Autodesk Fusion 360 part; units mm, degrees
sketch "Sketch1" plane through (0, 0, 0) normal (0, 0, 1) x (1, 0, 0) in component "Some Fidget Keyboard"
  line L0 (0, 0) -> (42.54, 0)
  line L1 (42.54, 0) -> (42.54, 62.204)
  line L2 (42.54, 62.204) -> (0, 62.204)
  line L3 (0, 62.204) -> (0, 0)
  line L4 (-9.5, 72.704) -> (53.04, 72.704)
  line L5 (53.04, 72.704) -> (53.04, -9.5)
  line L6 (53.04, -9.5) -> (-9.5, -9.5)
  line L7 (-9.5, -9.5) -> (-9.5, 72.704)
  circle A0 centre (-4.5, 67.704) radius 1.7
  circle A1 centre (48.04, 67.704) radius 1.7
  circle A2 centre (48.04, -4.5) radius 1.7
  circle A3 centre (-4.5, -4.5) radius 1.7
  circle A4 centre (-4.5, 67.704) radius 3
  circle A5 centre (48.04, 67.704) radius 3
  circle A6 centre (48.04, -4.5) radius 3
  circle A7 centre (-4.5, -4.5) radius 3
  dimension "d4" = 42.54
  dimension "d5" = 62.204
  dimension "d6" = 62.54
  dimension "d7" = 82.204
  dimension "d8" = 9.5
  dimension "d9" = 9.5
  dimension "d10" = 3.4
  dimension "d11" = 3.4
  dimension "d12" = 3.4
  dimension "d13" = 3.4
  dimension "d14" = 5
  dimension "d15" = 5
  dimension "d16" = 5
  dimension "d17" = 5
  dimension "d18" = 5
  dimension "d20" = 5
  dimension "d21" = 5
  dimension "d22" = 5
  dimension "d23" = 6
  dimension "d24" = 6
  dimension "d25" = 6
  dimension "d26" = 6
extrude "Extrude1" add sketch "Sketch1" along normal blind 9.9 from surface at 3.1 contours A4 | A5 | A6 | A7 makes body 1 at (45.4801, 66.1397, 9.7) makes body 2 at (-7.0599, 66.1397, 9.7) makes body 3 at (51.0363, -4.6495, 9.7) makes body 4 at (-1.5037, -4.6495, 9.7) in component "Some Fidget Keyboard"
extrude "Extrude2" add sketch "Sketch1" along normal blind 13 contours L4 L5 L6 L7 bodies 1 2 3 4 in component "Some Fidget Keyboard"
extrude "Extrude3" add sketch "Sketch1" along normal blind 3 contours L0 L1 L2 L3 bodies 1 in component "Some Fidget Keyboard"
sketch "Sketch2" plane through (0, 0, 0) normal (0, 0, 1) x (1, 0, 0) in component "Some Fidget Keyboard"
sketch "Sketch3" plane through (0, 0, 13) normal (0, 0, 1) x (-1, 0, 0) in component "Some Fidget Keyboard"
  circle A0 centre (-48.04, -67.704) radius 1.7
  circle A1 centre (4.5, 4.5) radius 1.7
  line L0 (0, 0) -> (0, -62.204)
  line L1 (0, -62.204) -> (-42.54, -62.204)
  line L2 (-42.54, -62.204) -> (-42.54, 0)
  line L3 (-42.54, 0) -> (0, 0)
  line L4 (9.5, 9.5) -> (-53.04, 9.5)
  line L5 (-53.04, 9.5) -> (-53.04, -72.704)
  line L6 (-53.04, -72.704) -> (9.5, -72.704)
  line L7 (9.5, -72.704) -> (9.5, 9.5)
  circle A2 centre (4.5, -67.704) radius 1.7
  circle A3 centre (-48.04, 4.5) radius 1.7
  line L8 (-30.93, 9.5) -> (-12.43, 9.5)
  line L9 (-12.43, 9.5) -> (-12.43, 0)
  line L10 (-12.43, 0) -> (-30.93, 0)
  line L11 (-30.93, 0) -> (-30.93, 9.5)
  line L12 (-53.04, -72.704) -> (-53.04, 9.5)
  dimension "d36" = 18.5
  dimension "d37" = 22.11
extrude "Extrude4" cut sketch "Sketch3" against normal blind 7.5 contours L3 L4 L8 L9 L10 L11 bodies 1 in component "Some Fidget Keyboard"
fillet "Fillet1" radius 5 1 edges at (-9.5, -9.5, 6.5) on bodies 1 in component "Some Fidget Keyboard"
fillet "Fillet2" radius 5 1 edges at (-9.5, 72.704, 6.5) on bodies 1 in component "Some Fidget Keyboard"
fillet "Fillet3" radius 5 2 edges at (53.04, 72.704, 6.5) (53.04, -9.5, 6.5) on bodies 1 in component "Some Fidget Keyboard"
sketch "Sketch1 (2)" plane through (0, 0, 0) normal (0, 0, 1) x (1, 0, 0)
sketch "Sketch2 (2)" plane through (0, 0, 3) normal (0, 0, 1) x (-1, 0, 0)
  line L0 (0, -62.204) -> (0, 0)
  line L1 (0, 0) -> (-42.54, 0)
  line L2 (-42.54, 0) -> (-42.54, -62.204)
  line L3 (-42.54, -62.204) -> (0, -62.204)
component "Some Fidget Keyboard" placed x (1, 0, 0) y (0, 1, 0) z (0, 0, 1) at (0, 0, 0)
Can you work these out from the model? Positions are in its coordinate system, mm. A direction names the side the tool comes from. Coordinates: 2 decimals unless noted, no trailing zeros. Loops run counter-clockwise (first coordinate to the right, second up) from the corner with the lowest first, then second, coordinate; pieces in that order, holes last. Notation, with made-up numbers: (-6, -31.5) - (13, -31.5) arc R27 cw to (13, -10.5) - close; hole circle Ø11 at (49.25, 87). An arc over 180 degrees is marked (long way). Put each result on its own line as item: value. Start each with the question number.
Item 1: Which directions (+Z, -Z, +X, -X, +Y, -Y) give clear straight access to the entire face, cutting with the end or side of a thin tool? Please do faces 1 (the face through (30.93, -5, 9)), 2 (the face through (0, 32, 8)), 3 (the face through (49.61, -3.85, 7.98)), 4 (the face through (-3, 66, 3.1)).
Item 2: Suppose I cut it at B-B (x = 5). Please give me the cut outline in (y, z).
Item 3: If I drill on line 1 along Y through (x, z) = (48.04, 1.85); line 2 along X through (y, z) = (49, 7.5); line 3 along Y through (x, z) = (35.5, 11.5), over which ranges is the centre line in solid material (lowest first)?
Item 4: Suppose I cut it at A-A (z = 10.75). Please give me the cut outline in (x, y).
Item 5: For pin 1 (4 mm diameter, centred on x = -4.5, y = 67.704, fed in from -Z); pin 2 (6 mm diameter, centred on x = 32.5, y = 41.5, fed in from +Z); pin 3 (7.5 mm diameter, centred on x = 22.5, y = -2.5, fed in from +Z), each with a flat end and sliding along its axis, tell me the tip position at first contact or that it passes through.
Item 6: If we mould it in two halves opening along Y, with no side actions, what happens to faces 5 (the face through (22, 62.204, 8)), 6 (the face through (-7.996, 71.278, 6.591)), 7 (the face through (-2, 38, 13))? For each: +Y half, -Y half, draft (parallel to the pull), parting line (faces both ways), or undercut.
Here are the results:
1. face 1: +Z, -Y
1. face 2: +Z
1. face 3: +Z, -Z
1. face 4: -Z
2. outline: (-9.5, 0) - (72.7, 0) - (72.7, 13) - (62.2, 13) - (62.2, 3) - (0, 3) - (0, 13) - (-9.5, 13) - close
3. line 1: -9.5 to -7.5, -1.5 to 64.7, 70.7 to 72.7
3. line 2: -9.5 to 0, 42.54 to 53.04
3. line 3: -9.5 to 0, 62.2 to 72.7
4. outline: (-9.5, -4.5) arc R5 ccw to (-4.5, -9.5) - (12.43, -9.5) - (12.43, 0) - (0, 0) - (0, 62.2) - (42.54, 62.2) - (42.54, 0) - (30.93, 0) - (30.93, -9.5) - (48.04, -9.5) arc R5 ccw to (53.04, -4.5) - (53.04, 67.7) arc R5 ccw to (48.04, 72.7) - (-4.5, 72.7) arc R5 ccw to (-9.5, 67.7) - close; hole circle Ø3.4 at (-4.5, -4.5); hole circle Ø3.4 at (-4.5, 67.7); hole circle Ø3.4 at (48.04, -4.5); hole circle Ø3.4 at (48.04, 67.7)
5. pin 1: z = 3.1
5. pin 2: z = 3
5. pin 3: z = 5.5
6. face 5: undercut
6. face 6: +Y half
6. face 7: draft
